from build123d import *

# Parameters (mm, degrees)
SKETCH1_W           = 189
SKETCH1_H           = 50
BOSS_EXTRUDE1_DEPTH = 1
SKETCH2_W           = 55
SKETCH2_H           = 18
CUT_EXTRUDE1_DEPTH  = 2
SKETCH3_W           = 2
SKETCH3_H           = 25
CUT_EXTRUDE2_DEPTH  = 2


with BuildPart() as part:
    # Sketch1 → Boss-Extrude1 (new body)
    with BuildSketch(Plane.XY):
        with Locations((32.8655586, 16.198012015)):
            Rectangle(SKETCH1_W, SKETCH1_H)
    extrude(amount=BOSS_EXTRUDE1_DEPTH)

    # Sketch2 → Cut-Extrude1 (cut, through all)
    with BuildSketch(Plane.XY.offset(1)):
        with Locations((49.8655586, 2.198012015)):
            Rectangle(SKETCH2_W, SKETCH2_H)
    extrude(amount=-CUT_EXTRUDE1_DEPTH, mode=Mode.SUBTRACT)

    # Sketch3 → Cut-Extrude2 (cut, through all)
    with BuildSketch(Plane(origin=(0, 0, 0), x_dir=(-1, 0, 0), z_dir=(0, 0, -1))):
        with Locations((-11.3655586, 16.198012015)):
            Rectangle(SKETCH3_W, SKETCH3_H)
        with Locations((-7.3655586, 16.198012015)):
            Rectangle(SKETCH3_W, SKETCH3_H)
        with Locations((-3.3655586, 16.198012015)):
            Rectangle(SKETCH3_W, SKETCH3_H)
        with Locations((0.6344414, 16.198012015)):
            Rectangle(SKETCH3_W, SKETCH3_H)
        with Locations((4.6344414, 16.198012015)):
            Rectangle(SKETCH3_W, SKETCH3_H)
        with Locations((8.6344414, 16.198012015)):
            Rectangle(SKETCH3_W, SKETCH3_H)
        with Locations((12.6344414, 16.198012015)):
            Rectangle(SKETCH3_W, SKETCH3_H)
        with Locations((16.6344414, 16.198012015)):
            Rectangle(SKETCH3_W, SKETCH3_H)
        with Locations((20.6344414, 16.198012015)):
            Rectangle(SKETCH3_W, SKETCH3_H)
        with Locations((24.6344414, 16.198012015)):
            Rectangle(SKETCH3_W, SKETCH3_H)
        with Locations((28.6344414, 16.198012015)):
            Rectangle(SKETCH3_W, SKETCH3_H)
        with Locations((32.6344414, 16.198012015)):
            Rectangle(SKETCH3_W, SKETCH3_H)
        with Locations((36.6344414, 16.198012015)):
            Rectangle(SKETCH3_W, SKETCH3_H)
        with Locations((40.6344414, 16.198012015)):
            Rectangle(SKETCH3_W, SKETCH3_H)
        with Locations((44.6344414, 16.198012015)):
            Rectangle(SKETCH3_W, SKETCH3_H)
    extrude(amount=-CUT_EXTRUDE2_DEPTH, mode=Mode.SUBTRACT)


solid = part.part
The listing builds one solid part. Answer for the finished solid, in the listing's coordinates (mm). Coordinates: 2 decimals unless noted, no trailing zeros. Order: outer loops, then holes, each group sorted by start corner. A loop starts at its lowest first (then second) coordinate and runs counter-clockwise, first axis right, second up. Notation, with made-up numbers: (58.5, 85.5) -> (77.5, 85.5) arc R30 cw to (77.5, 123.5) -> close; hole circle Ø9 at (34, 44.25). An arc over 180 degrees is marked (long way). Answer in a Markdown table with one row per item. Add a question column.
Item 1: Find section B-B (y = -3). Write down the section's boundary in (x, z), then the cut area to 3 significant figures.
Item 2: Find section A-A (x = 53). Write down the section's boundary in (y, z), then the cut area to 3 significant figures.
Item 3: Find the intervals of material crossed by L1, parallel to Y at x = 46, z = 0.35; L2, parallel to Y at x = -44.5, z = 0.2; L3, parallel to X at y = -4, z = 0.7, in increasing order. Write a range as from..to.
Item 4: This flat-tipped pin is pushed along its axis until it touches: P1, Ø1.5, axis at x = 6, y = 24.5, coming from the -Z side. Where does it stop, or does it pass through?
Item 5: Find section C-C (y = 8). State how many separate pieces and enclosed holes the cut face has, then the cut area to 3 significant figures.
Result set:
| question | item | result |
|---|---|---|
| 1 | outline | (-61.63, 0) -> (22.37, 0) -> (22.37, 1) -> (-61.63, 1) -> close; (77.37, 0) -> (127.37, 0) -> (127.37, 1) -> (77.37, 1) -> close |
| 1 | area | 134 mm² |
| 2 | outline | (-8.8, 0) -> (-6.8, 0) -> (-6.8, 1) -> (-8.8, 1) -> close; (11.2, 0) -> (41.2, 0) -> (41.2, 1) -> (11.2, 1) -> close |
| 2 | area | 32.0 mm² |
| 3 | L1 | y = -8.8..-6.8, 11.2..41.2 |
| 3 | L2 | y = -8.8..3.7, 28.7..41.2 |
| 3 | L3 | x = -61.63..22.37, 77.37..127.37 |
| 4 | P1 | stops at z = 0 |
| 5 | separate pieces | 17 |
| 5 | enclosed holes | 0 |
| 5 | area | 104 mm² |
